```python
from build123d import *

# Parameters (mm, degrees)
F1_DEPTH = 75
F3_DEPTH = 20
F5_DEPTH = 59.331604


with BuildPart() as f1:
    # F0 (on Top) → F1 (new body)
    with BuildSketch(Plane.XY):
        with BuildLine():
            Line((0, 26.765937), (-54.154223, 12.255357))
            Line((-54.154223, 12.255357), (-54.154223, -27.744643))
            Line((-54.154223, -27.744643), (-39.154223, -27.744643))
            Line((-39.154223, -27.744643), (-39.154223, -13.744643))
            ThreePointArc((-39.154223, -13.744643), (-29.306659, -4.077686), (-19.823619, -14.102482))
            Line((-19.823619, -14.102482), (-19.823619, -27.626852))
            Line((-19.823619, -27.626852), (5.176381, -27.626852))
            Line((5.176381, -27.626852), (5.176381, -2.626852))
            Line((5.176381, -2.626852), (25.176381, -2.626852))
            Line((25.176381, -2.626852), (25.176381, 7.44742))
            ThreePointArc((25.176381, 7.44742), (17.351609, 23.314487), (0, 26.765937))
        make_face()
    extrude(amount=F1_DEPTH)

    # F2 (on face) → F3 (join)
    with BuildSketch(Plane.XY.offset(75)):
        with BuildLine():
            ThreePointArc((21.116702, 19.526583), (-2.439619, 7.072345), (23.856985, 11.373148))
            ThreePointArc((23.856985, 11.373148), (23.15359, 15.673952), (21.116702, 19.526583))
        make_face()
    extrude(amount=F3_DEPTH)

    # F4 (on face) → F5 (cut, through all)
    with BuildSketch(Plane.YZ.offset(5.176381)):
        Polygon((-7.626852, 0), (-27.626852, 20), (-27.626852, 0), align=None)
        Polygon((-7.626852, 45), (-27.626852, 55), (-27.626852, 42.03419), align=None)
    extrude(amount=-F5_DEPTH, mode=Mode.SUBTRACT)


solid = f1.part
```
Input: part model. Units: mm. Frame: model coordinates. A direction names the side the tool comes from. Coordinates: 2 decimals unless noted, no trailing zeros. Order: outer loops, then holes, each group sorted by start corner. A loop starts at its lowest first (then second) coordinate and runs counter-clockwise, first axis right, second up. Notation, with made-up numbers: (30.25, -15.5) - (34.25, -15.5) arc R16 cw to (34.25, -4.5) - close; hole circle Ø3 at (11.5, 44). An arc over 180 degrees is marked (long way). Return JSON: item names as keys, results as strings.
Q1. Cut plane D-D (z = 36.5). Return loops of the section in (x, y).
The answers:
{"outline": "(-54.15, -27.74) - (-39.15, -27.74) - (-39.15, -13.74) arc R9.67 cw (long way) to (-19.82, -14.1) - (-19.82, -27.63) - (5.18, -27.63) - (5.18, -2.63) - (25.18, -2.63) - (25.18, 7.45) arc R20 ccw to (0, 26.77) - (-54.15, 12.26) - close"}
Q2. Draft query along X for faces 1 (the flat face through (-47, -27.745, 37)), 2 (the flat face through (-39.154, -21, 37)), 3 (the flat face through (-54.154, -7, 37)). Return one class per face: +X half, -X half, draft (parallel to the pull), parting line (faces both ways), or undercut.
The answers:
{"face 1": "draft", "face 2": "undercut", "face 3": "-X half"}
Q3. Cut plane B-B (y = -20). Return loops of the section in (x, z).
The answers:
{"outline": "(-54.15, 12.37) - (-39.15, 12.37) - (-39.15, 43.17) - (-54.15, 43.17) - close; (-54.15, 51.19) - (-39.15, 51.19) - (-39.15, 75) - (-54.15, 75) - close; (-19.82, 12.37) - (5.18, 12.37) - (5.18, 43.17) - (-19.82, 43.17) - close; (-19.82, 51.19) - (5.18, 51.19) - (5.18, 75) - (-19.82, 75) - close"}
Q4. Cut plane C-C (x = -8). Return loops of the section in (y, z), then the cut area to 3 significant figures.
The answers:
{"outline": "(-27.63, 20) - (-7.63, 0) - (24.62, 0) - (24.62, 75) - (-27.63, 75) - (-27.63, 55) - (-7.63, 45) - (-27.63, 42.03) - close", "area": "3,590 mm2"}
Q5. Cut plane A-A (z = 9). Return loops of the section in (x, y).
The answers:
{"outline": "(-54.15, -27.74) - (-39.15, -27.74) - (-39.15, -27.63) - (-54.15, -27.63) - close; (-54.15, -16.63) - (-39.15, -16.63) - (-39.15, -13.74) arc R9.67 cw (long way) to (-19.82, -14.1) - (-19.82, -16.63) - (5.18, -16.63) - (5.18, -2.63) - (25.18, -2.63) - (25.18, 7.45) arc R20 ccw to (0, 26.77) - (-54.15, 12.26) - close"}
Q6. First-contact query: pin 1 (10 mm diameter, centred on x = 19, z = 30.5, fed in from -Y); pin 2 (5 mm diameter, centred on x = -20, z = 49.5, fed in from +Y); pin 3 (8 mm diameter, centred on y = -21.5, z = 36.5, fed in from +X). Flat tips, straight axial feed; report the tip coordinate or a pass-through.
The answers:
{"pin 1": "stops at y = -2.63", "pin 2": "stops at y = 22.08", "pin 3": "stops at x = 5.18"}
Q7. Ray query, probe 1 along X at (y, z) = (-3, 19); probe 2 along X at (y, z) = (-8, 65.5); probe 3 along X at (y, z) = (-23, 64). Return the intervals inside material, ascending.
The answers:
{"probe 1": "x = -54.15 to 5.18", "probe 2": "x = -54.15 to -37.26, -21.71 to 5.18", "probe 3": "x = -54.15 to -39.15, -19.82 to 5.18"}
Q8. Access query for faces 4 (the flat face through (-19.824, -21, 64)), 5 (the flat face through (15, -2.627, 37)), 6 (the flat face through (-26.7, 19.61, 36.98)), 7 (the flat face through (-45.443, -17.487, 9.86)). Directions: +Z, -Z, +X, -X, +Y, -Y. A direction counts if a zero-diameter tool reaches every point of the face in a straight line with its end or side. Return the directions, or none.
The answers:
{"face 4": "+Z, -Z, -Y", "face 5": "+Z, -Z, +X, -Y", "face 6": "+Z, -Z, -X, +Y", "face 7": "-Z, +X, -X"}
